```python
from build123d import *

# Parameters (mm, degrees)
SKETCH1_R               = 22
BOSS_EXTRUDE1_DEPTH     = 10
SKETCH2_R               = 12.5
BOSS_EXTRUDE2_DEPTH     = 6
CUT_EXTRUDE1_REACH      = 36.986
CUT_EXTRUDE1_END_RADIUS = 12.5
SKETCH3_R               = 1.5
CUT_EXTRUDE2_REACH      = 36.986
SKETCH4_R               = 4
CUT_EXTRUDE3_START      = -1.33
SKETCH5_R               = 22
SKETCH5_R_2             = 19
CUT_EXTRUDE3_DEPTH      = 7.33333
CHAMFER1_SIZE           = 2
CHAMFER1_SIZE_2         = 0.666
CHAMFER2_SIZE           = 0.5


with BuildPart() as part:
    # Sketch1 → Boss-Extrude1 (new body)
    with BuildSketch(Plane(origin=(0, 0, 0), x_dir=(1, 0, 0), z_dir=(0, 1, 0))):
        with Locations(Location((0, 0, 0), (0, 0, 270))):
            Circle(SKETCH1_R)
    extrude(amount=BOSS_EXTRUDE1_DEPTH)

    # Sketch2 → Boss-Extrude2 (add)
    with BuildSketch(Plane(origin=(0, 10, 0), x_dir=(1, 0, 0), z_dir=(0, 1, 0))):
        with Locations(Location((0, 0, 0), (0, 0, 270))):
            Circle(SKETCH2_R)
    extrude(amount=BOSS_EXTRUDE2_DEPTH)

    # Cut-Extrude1: up to this cylinder (the profile starts inside it)
    cut_extrude1_end = Plane(origin=(0, 13, 0), z_dir=(0, -1, 0)) * Cylinder(CUT_EXTRUDE1_END_RADIUS, 99.972, mode=Mode.PRIVATE)
    # Sketch3 → Cut-Extrude1 (cut, up to the surface)
    with BuildSketch(Plane.XY, mode=Mode.PRIVATE) as cut_extrude1_sk1:
        with Locations((0, 13)):
            Circle(SKETCH3_R)
    cut_extrude1_tool1 = extrude(cut_extrude1_sk1.sketch, amount=-CUT_EXTRUDE1_REACH, mode=Mode.PRIVATE) & cut_extrude1_end
    add(cut_extrude1_tool1.solids().sort_by_distance((0, 13, 0))[0], mode=Mode.SUBTRACT)

    # Sketch4 → Cut-Extrude2 (cut, up to next)
    with BuildSketch(Plane(origin=(0, 16, 0), x_dir=(1, 0, 0), z_dir=(0, 1, 0)), mode=Mode.PRIVATE) as cut_extrude2_sk1:
        with Locations(Location((0, 0, 0), (0, 0, 270))):
            Circle(SKETCH4_R)
    cut_extrude2_tool1 = extrude(cut_extrude2_sk1.sketch, amount=-CUT_EXTRUDE2_REACH, mode=Mode.PRIVATE) & part.part
    add(cut_extrude2_tool1.solids().sort_by_distance((0, 16, 0))[0], mode=Mode.SUBTRACT)

    # Sketch5 → Cut-Extrude3 (cut)
    with BuildSketch(Plane.XZ.offset(CUT_EXTRUDE3_START)):
        with Locations(Location((0, 0, 0), (0, 0, 270))):
            Circle(SKETCH5_R)
        with Locations(Location((0, 0, 0), (0, 0, 270))):
            Circle(SKETCH5_R_2, mode=Mode.SUBTRACT)
    extrude(amount=-CUT_EXTRUDE3_DEPTH, mode=Mode.SUBTRACT)

    # Chamfer1
    # the kernel refuses this chamfer: 2, 0.666 mm, written as the material it takes off along each edge
    with BuildSketch(Plane(origin=(0, 1.33, 0), x_dir=(0, 0, 1), z_dir=(1, 0, 0))) as chamfer1_piece_1:
        Polygon((22, CHAMFER1_SIZE), (22 - CHAMFER1_SIZE_2, 0), (22, 0), align=None)
    revolve(axis=Axis((0, 1.33, 0), (0, -1, 0)), mode=Mode.SUBTRACT)
    with BuildSketch(Plane(origin=(0, 8.66333, 0), x_dir=(0, 0, 1), z_dir=(1, 0, 0))) as chamfer1_piece_2:
        Polygon((22 - CHAMFER1_SIZE, 0), (22, -CHAMFER1_SIZE_2), (22, 0), align=None)
    revolve(axis=Axis((0, 8.66333, 0), (0, -1, 0)), mode=Mode.SUBTRACT)

    # Chamfer2
    chamfer2_edges = [part.edges().sort_by_distance(p)[0] for p in [
        (0, 16, -4),
        (0, 0, -4),
        (0, 16, -12.5),
    ]]
    chamfer(chamfer2_edges, length=CHAMFER2_SIZE)


solid = part.part
```
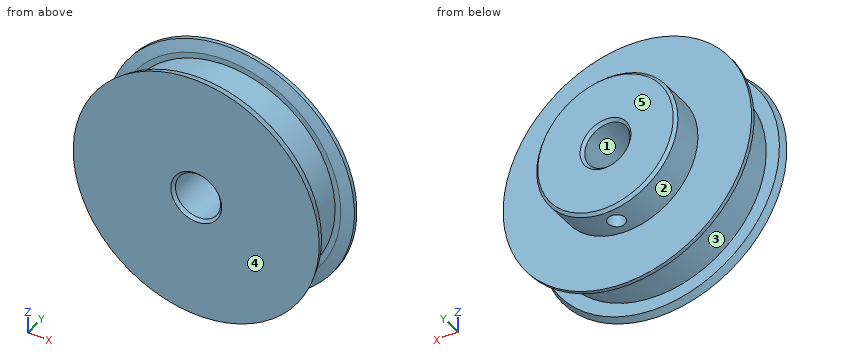
Work out the finished part from the listing and answer in its coordinate system (mm). Face numbers are marked on the shaded views. A direction names the side the tool comes from. Give positions to 0.01 mm unless a question says otherwise; leave off trailing zeros. Loops run counter-clockwise (first coordinate to the right, second up) from the corner with the lowest first, then second, coordinate; pieces in that order, holes last. Notation, with made-up numbers: M 81,83 L 97,83 A23 cw 97,100 Z; hole C 85,84 d6. An arc over 180 degrees is marked long. One line per item, written item: value. Start each with the question number.
1. Determine the mould class of the marked faces 3, 4 and 5 for opening direction Y: released by +Y, released by -Y, zero draft, split by the parting line, or undercut.
2. Each of these flat-tipped pins is pushed along its axis until it touches: P1, Ø3, axis at y = 13.5, z = -6.5, coming from the -X side; P2, Ø5, axis at x = 15, y = 3.5, coming from the -Z side; P3, Ø4, axis at x = 0, y = 13, coming from the -Z side. Where does it stop, or does it pass through?
3. Find section A-A (z = 0). Give the vertices of the cut face in (x, y), and give its area (3 significant figures).
4. Find section D-D (y = 13). Give the vertices of the cut face in (x, z).
5. Find section C-C (y = 4). Give the vertices of the cut face in (x, z), and give its area (3 significant figures).
6. Find the intervals of material crossed by probe 1 along X at (y, z) = (9.75, 0); probe 2 along Y at (x, z) = (15.5, -3.5); probe 3 along Z at (x, y) = (-1.5, 15), in increasing order.
7. Find section B-B (x = 0). State how many separate pieces and enclosed holes the cut face has, and give its area (3 significant figures).
8. Which of the six approach directions +Z, -Z, +X, -X, +Y, -Y give full straight-line access (tool end or side, diameter ignored) to the marked faces 1 and 2?
Reported:
1. face 3: undercut
1. face 4: released by -Y
1. face 5: released by +Y
2. P1: stops at x = -11.46
2. P2: stops at z = -16.3
2. P3: stops at z = -12.5
3. outline: M -22,9.33 L -20,8.66 L -19,8.66 L -19,1.33 L -21.33,1.33 L -21.78,0 L -4.5,0 L -4,0.5 L -4,15.5 L -4.5,16 L -12,16 L -12.5,15.5 L -12.5,10 L -22,10 Z; M 4,0.5 L 4.5,0 L 21.78,0 L 21.33,1.33 L 19,1.33 L 19,8.66 L 20,8.66 L 22,9.33 L 22,10 L 12.5,10 L 12.5,15.5 L 12,16 L 4.5,16 L 4,15.5 Z
3. area: 415 mm²
4. outline: M -1.5,-12.41 L -1.5,-3.71 A4 cw long 1.5,-3.71 L 1.5,-12.41 A12.5 ccw long Z
5. outline: C 0,0 d38; hole C 0,0 d8
5. area: 1,080 mm²
6. probe 1: x = -22 to -4, 4 to 22
6. probe 2: y = 0 to 10
6. probe 3: z = -12.41 to -3.71, 3.71 to 12.41
7. separate pieces: 3
7. enclosed holes: 0
7. area: 389 mm²
8. face 1: +Y, -Y
8. face 2: +Y
